For this review, take the finished solid that the model builds, in its own axes (mm). A direction names the side the tool comes from. Round coordinates to 2 decimals unless told otherwise and drop trailing zeros. Order: outer loops, then holes, each group sorted by start corner. A loop starts at its lowest first (then second) coordinate and runs counter-clockwise, first axis right, second up. Notation, with made-up numbers: (68.5, 28) -> (116.5, 28) arc R13 ccw to (116.5, 45) -> close; hole circle Ø6 at (-31.5, 30.25). An arc over 180 degrees is marked (long way). Put each result on its own line as item: value. Start each with the question number.
```python
from build123d import *

# Parameters (mm, degrees)
PAD003_DEPTH      = 2
BOX005_W          = 112
BOX005_H          = 51.4
BOX005_DEPTH      = 10
BOX004_W          = 118
BOX004_H          = 57.4
BOX004_DEPTH      = 10
PAD004_DEPTH      = 3
ARRAY001_X_COUNT  = 2
ARRAY001_X_PITCH  = 17
CYLINDER001_R     = 4
CYLINDER001_DEPTH = 30
CYLINDER_R        = 2.2
CYLINDER_DEPTH    = 30
BOX006_W          = 20
BOX006_H          = 5
BOX006_DEPTH      = 30
BOX007_W          = 6
BOX007_H          = 4
BOX007_DEPTH      = 10
PAD002_DEPTH      = 10


with BuildPart() as body003:
    # Sketch003 → Pad003 (new body)
    with BuildSketch(Plane.XY):
        Polygon((-59, -28.7), (-44.857864, -28.7), (-59, -14.557864), align=None)
    extrude(amount=PAD003_DEPTH)


with BuildPart() as part_mirroring001:
    # Part__Mirroring001: instance of Body003
    add(body003.part.mirror(Plane(origin=(0, 0, 0), x_dir=(1, 0, 0), z_dir=(0, 1, 0))))


with BuildPart() as fusion005:
    # Fusion005 base: copy of Body003
    add(body003.part)

    # Fusion005: union Part__Mirroring001
    add(part_mirroring001.part)


with BuildPart() as corners_fusion:
    # Part__Mirroring002: instance of Fusion005
    add(fusion005.part.mirror(Plane(origin=(0, 0, 0), x_dir=(0, -1, 0), z_dir=(1, 0, 0))))

    # Fusion006: union Fusion005
    add(fusion005.part)


with BuildPart() as corners_fusion_1:
    # Fusion006 placement: moved
    add(corners_fusion.part.moved(Location((0, 0, 8))))


with BuildPart() as middle_pocket_cube:
    # Box005 → Box005 (new body)
    with BuildSketch(Plane(origin=(-56, -25.7, 0), x_dir=(1, 0, 0), z_dir=(0, 0, 1))):
        with Locations((56, 25.7)):
            Rectangle(BOX005_W, BOX005_H)
    extrude(amount=BOX005_DEPTH)


with BuildPart() as middle_external:
    # Box004 → Box004 (new body)
    with BuildSketch(Plane(origin=(-59, -28.7, 0), x_dir=(1, 0, 0), z_dir=(0, 0, 1))):
        with Locations((59, 28.7)):
            Rectangle(BOX004_W, BOX004_H)
    extrude(amount=BOX004_DEPTH)


with BuildPart() as triangles_array:
    # Sketch004 → Pad004 (new body)
    with BuildSketch(Plane.YZ):
        Polygon((41.5, 30), (27.205015, 8.579618), (41.5, 0), align=None)
    extrude(amount=PAD004_DEPTH)

    # Array001 X: triangles array ×2


with BuildPart() as triangles_array_1:
    add(triangles_array.part)
    with Locations(*[(i * ARRAY001_X_PITCH, 0, 0) for i in range(1, ARRAY001_X_COUNT)]):
        add(triangles_array.part)


with BuildPart() as triangles_array_2:
    # Array001 placement: moved
    add(triangles_array_1.part.moved(Location((-10, 0, 0))))


with BuildPart() as bolt_head_hole:
    # Cylinder001 → Cylinder001 (new body)
    with BuildSketch(Plane.XZ.offset(14)):
        Circle(CYLINDER001_R)
    extrude(amount=CYLINDER001_DEPTH)


with BuildPart() as bolt_fusion_clone:
    # Cylinder → Cylinder (new body)
    with BuildSketch(Plane.XZ):
        Circle(CYLINDER_R)
    extrude(amount=CYLINDER_DEPTH)

    # Fusion002: union bolt head hole
    add(bolt_head_hole.part)


with BuildPart() as bolt_fusion_clone_1:
    # Body005 placement: moved
    add(bolt_fusion_clone.part.moved(Location((0, 57, 21))))


with BuildPart() as middle_attach_cube:
    # Box006 → Box006 (new body)
    with BuildSketch(Plane(origin=(-10, 0, 0), x_dir=(1, 0, 0), z_dir=(0, 0, 1))):
        with Locations((10, 2.5)):
            Rectangle(BOX006_W, BOX006_H)
    extrude(amount=BOX006_DEPTH)


with BuildPart() as middle_attach_cut:
    # Box007 → Box007 (new body)
    with BuildSketch(Plane(origin=(-3, 5, 0), x_dir=(1, 0, 0), z_dir=(0, 0, 1))):
        with Locations((3, 2)):
            Rectangle(BOX007_W, BOX007_H)
    extrude(amount=BOX007_DEPTH)

    # Fusion008: union middle attach cube
    add(middle_attach_cube.part)


with BuildPart() as middle_attach_cut_1:
    # Fusion008 placement: moved
    add(middle_attach_cut.part.moved(Location((0, 41.7, 0))))

    # Cut002: cut bolt fusion clone
    add(bolt_fusion_clone_1.part, mode=Mode.SUBTRACT)


with BuildPart() as middle_with_corners:
    # Sketch002 → Pad002 (new body)
    with BuildSketch(Plane.XY):
        with BuildLine():
            Line((-59, 28.7), (59, 28.7))
            Line((59, 28.7), (23.942659, 43.821249))
            ThreePointArc((23.942659, 43.821249), (17.118373, 45.972801), (10, 46.7))
            Line((10, 46.7), (-10, 46.7))
            ThreePointArc((-10, 46.7), (-17.118373, 45.972801), (-23.942659, 43.821249))
            Line((-23.942659, 43.821249), (-59, 28.7))
        make_face()
    extrude(amount=PAD002_DEPTH)

    # Fusion004: union middle external, triangles array, middle attach cut
    add(middle_external.part)
    add(triangles_array_2.part)
    add(middle_attach_cut_1.part)

    # Cut: cut middle pocket cube
    add(middle_pocket_cube.part, mode=Mode.SUBTRACT)

    # Fusion007: union corners fusion
    add(corners_fusion_1.part)


solid = middle_with_corners.part
```
Item 1: Consider section D-D, the plane x = -31. Write out the cut boundary in (y, z).
Item 2: Mouldability with a two-part tool opening along Y and no side actions: class faces 4 (the face through (-51.87, -21.69, 8.99)), 5 (the face through (2, 43, 19)), 6 (the face through (-41.226, 36.366, 4.93)) as +Y half, -Y half, draft (parallel to the pull), parting line (faces both ways), or undercut.
Item 3: Tool access review of faces 1 (the face through (10, 38, 16)), 2 (the face through (-9, 41.5, 20)), 3 (the face through (-1, -25.7, 5)): name each direction out of +Z, -Z, +X, -X, +Y, -Y from which nothing blocks a thin tool from reaching the whole face with its end or side.
Item 4: Consider section B-B, the plane z = 14. Write out the cut boundary in (x, y), plus the area to 3 significant figures.
Item 5: Consider section C-C, the plane x = 0. Write out the cut boundary in (y, z), plus the area to 3 significant figures.
Item 6: Consider section A-A, the plane y = 7. Write out the cut boundary in (x, z).
Item 7: For L1, parallel to X at y = 17, z = 9.25; L2, parallel to Z at x = 0, y = 42.3; L3, parallel to X at y = 45.6, z = 21, list the stretches that pass through material, from the lowest coordinate up.
Item 8: Insertion check: pin 1 Ø3 at (y, z) = (36, 17.5) entering from +X; pin 2 Ø2.5 at (x, y) = (-53.5, -22) entering from -Z; pin 3 Ø11 at (x, z) = (26, 4.5) entering from +Y; pin 4 Ø4 at (x, z) = (0, 21) entering from +Y. Each pin has a flat end and moves straight along its axis. Give the tip position at first contact, or say it passes through.
Evaluation:
1. outline: (-28.7, 0) -> (-25.7, 0) -> (-25.7, 10) -> (-28.7, 10) -> close; (25.7, 0) -> (40.78, 0) -> (40.78, 10) -> (25.7, 10) -> close
2. face 4: undercut
2. face 5: -Y half
2. face 6: +Y half
3. face 1: +Z, +X, +Y, -Y
3. face 2: +Z, +X, -X
3. face 3: -Z
4. outline: (-10, 30.82) -> (-7, 30.82) -> (-7, 41.5) -> (-10, 41.5) -> close; (-10, 41.7) -> (10, 41.7) -> (10, 46.7) -> (-10, 46.7) -> close; (7, 30.82) -> (10, 30.82) -> (10, 41.5) -> (7, 41.5) -> close
4. area: 164 mm^2
5. outline: (-28.7, 0) -> (-25.7, 0) -> (-25.7, 10) -> (-28.7, 10) -> close; (25.7, 0) -> (50.7, 0) -> (50.7, 10) -> (46.7, 10) -> (46.7, 18.8) -> (43, 18.8) -> (43, 17) -> (41.7, 17) -> (41.7, 10) -> (25.7, 10) -> close; (41.7, 25) -> (43, 25) -> (43, 23.2) -> (46.7, 23.2) -> (46.7, 30) -> (41.7, 30) -> close
5. area: 353 mm^2
6. outline: (-59, 0) -> (-56, 0) -> (-56, 10) -> (-59, 10) -> close; (56, 0) -> (59, 0) -> (59, 10) -> (56, 10) -> close
7. L1: x = -59 to -56, 56 to 59
7. L2: z = 0 to 17, 25 to 30
7. L3: x = -10 to -2.2, 2.2 to 10
8. pin 1: stops at x = 10
8. pin 2: stops at z = 8
8. pin 3: stops at y = 45.1
8. pin 4: passes through
